Verification items for the finished model (mm, model axes). Face numbers are marked on the shaded views. A direction names the side the tool comes from. Coordinates: 2 decimals unless noted, no trailing zeros. Order: outer loops, then holes, each group sorted by start corner. A loop starts at its lowest first (then second) coordinate and runs counter-clockwise, first axis right, second up. Notation, with made-up numbers: (-2.5, 69.5) - (35.5, 69.5) arc R31 cw to (35.5, 103.5) - close; hole circle Ø10 at (-40, 22). An arc over 180 degrees is marked (long way). Answer as CSV lines item,"result". Start each with the question number.
1. Section check C-C (y = 277.5). Record the cut outline in (x, z).
2. Go/stop test with flat-tipped pins: pin 1 (3 mm diameter, centred on x = -61.5, y = 284.5, fed in from -Z); pin 2 (1 mm diameter, centred on x = -444, y = 530, fed in from +Z); pin 3 (6 mm diameter, centred on y = 48, z = 742.5, fed in from -X). Record where each tip stops, or that it passes through.
3. Set-up check for the marked faces 1, 2 and 3: record each of +Z, -Z, +X, -X, +Y, -Y from which the full face is reachable in a straight line by a thin tool's end or side.
4. Mould release check, pull along Y, two halves, no side actions. Record for the marked faces 4, 5, 6 and 7: pulls with the +Y half, pulls with the -Y half, needs draft (parallel to the pull), parting line crosses it, or undercut.
5. Section check D-D (x = 46). Record the cut outline in (y, z).
6. Section check A-A (z = 166). Record the cut outline in (x, y).
7. Material ranges on L1, parallel to Y at x = -168.5, z = 90.5; L2, parallel to X at y = 134, z = 358; L3, parallel to Y at x = -249, z = 269.5, recorded low to high. Write a range as [from, to].
8. Section check B-B (x = -195). Record the cut outline in (y, z).
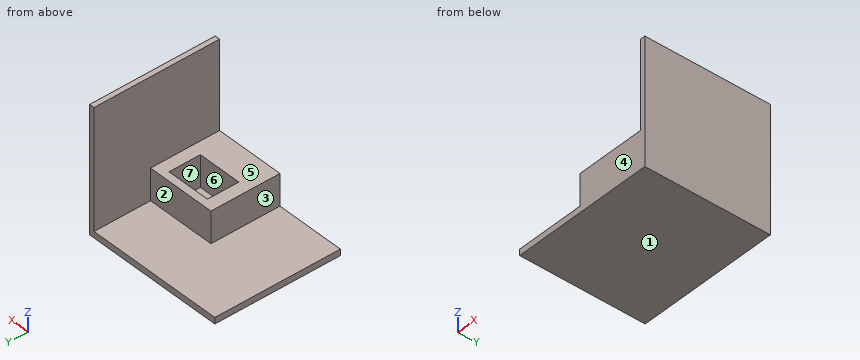
Autodesk Inventor part; units mm, degrees
ref_plane "YZ Plane" through (0, 0, 0) normal (1, 0, 0) x (0, 1, 0)
ref_plane "XZ Plane" through (0, 0, 0) normal (0, 1, 0) x (-1, 0, 0)
ref_plane "XY Plane" through (0, 0, 0) normal (0, 0, 1) x (1, 0, 0)
sketch "Boceto1" plane through (0, 0, 0) normal (0, 0, 1) x (1, 0, 0)
  line L0 (175, -125) -> (-175, -125)
  line L1 (-175, -125) -> (-175, 125)
  line L2 (-175, 125) -> (175, 125)
  line L3 (175, 125) -> (175, -125)
  line L4 (175, -125) -> (-175, 125) construction
  line L5 (-175, -125) -> (175, 125) construction
  line L6 (-175, 125) -> (-165, 125) construction
  line L7 (-175, 125) -> (-275, 125)
  line L8 (-275, 125) -> (-275, 185)
  line L9 (-275, 185) -> (-175, 185)
  line L10 (-175, 185) -> (-175, 125)
  line L11 (-275, 185) -> (275, 185)
  line L12 (275, 185) -> (275, -365)
  line L13 (275, -365) -> (-275, -365)
  line L14 (-275, -365) -> (-275, 185)
  point P0 (0, 0)
  dimension "d0" = 350
  dimension "d1" = 250
  dimension "d4" = 100
  dimension "d5" = 60
  dimension "d6" = 550
  dimension "d7" = 550
extrude "Extrusión1" add sketch "Boceto1" along normal blind 300
extrude "Extrusión2" add sketch "Boceto1" along normal blind 49 contours L0 L1 L2 L3
sketch "Boceto2" plane through (-275, -365, 0) normal (-1, 0, 0) x (0, 0, 1)
  line L0 (0, 550) -> (0, 0)
  line L1 (0, 0) -> (50, 0)
  line L2 (50, 0) -> (50, 1000)
  line L3 (50, 1000) -> (0, 1000)
  line L4 (0, 1000) -> (0, 0)
  point P0 (0, 365)
  dimension "d12" = 50
  dimension "d13" = 1000
extrude "Extrusión3" add sketch "Boceto2" along normal mid plane 1100
sketch "Boceto3" plane through (275, -365, 300) normal (1, 0, 0) x (0, 0, -1)
  line L0 (300, 0) -> (300, 1000)
  line L1 (300, 0) -> (-700, 0)
  line L2 (-700, 0) -> (-700, 1000)
  line L3 (-700, 1000) -> (300, 1000)
  line L4 (300, 1000) -> (300, 0)
  point P0 (300, 365)
  dimension "d16" = 1000
extrude "Extrusión4" add sketch "Boceto3" along normal blind 40
Evaluation:
1,outline,"(-825, 0) - (315, 0) - (315, 1000) - (275, 1000) - (275, 50) - (-825, 50) - close"
2,pin 1,"stops at z = 0"
2,pin 2,"stops at z = 50"
2,pin 3,"stops at x = 275"
3,face 1,"-Z, +X, -X, +Y, -Y"
3,face 2,"+Z, -X, +Y"
3,face 3,"+Z, -X, +Y, -Y"
4,face 4,"pulls with the -Y half"
4,face 5,"needs draft"
4,face 6,"undercut"
4,face 7,"undercut"
5,outline,"(-365, 0) - (635, 0) - (635, 50) - (185, 50) - (185, 300) - (125, 300) - (125, 50) - (-125, 50) - (-125, 300) - (-365, 300) - close"
6,outline,"(-275, -365) - (315, -365) - (315, 635) - (275, 635) - (275, 185) - (-275, 185) - close; hole (-175, -125) - (175, -125) - (175, 125) - (-175, 125) - close"
7,L1,"y = [-365, -125], [125, 185]"
7,L2,"x = [275, 315]"
7,L3,"y = [-365, 185]"
8,outline,"(-365, 0) - (635, 0) - (635, 50) - (185, 50) - (185, 300) - (-365, 300) - close"
